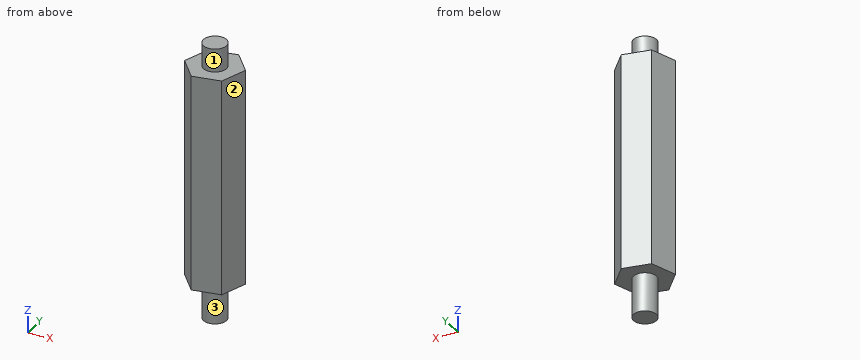
```python
from build123d import *

# Parameters (mm, degrees)
F0_R     = 1.5
F1_DEPTH = 28
F2_DEPTH = 5
F3_R     = 1.5
F4_DEPTH = 3


with BuildPart() as f1:
    # F0 (on Top) → F1 (new body)
    with BuildSketch(Plane.XY):
        Polygon((2.413244, -2.721443), (3.563461, 0.729209), (1.150217, 3.450652), (-2.413244, 2.721443), (-3.563461, -0.729209), (-1.150217, -3.450652), align=None)
        Circle(F0_R, mode=Mode.SUBTRACT)
        Circle(F0_R)
    extrude(amount=F1_DEPTH)

    # F0 (on Top) → F2 (join)
    with BuildSketch(Plane.XY):
        Circle(F0_R)
    extrude(amount=-F2_DEPTH)

    # F3 (on face) → F4 (join)
    with BuildSketch(Plane.XY.offset(28)):
        Circle(F3_R)
    extrude(amount=F4_DEPTH)


solid = f1.part
```
Design review of the part built by this model. Coordinates are the model's own, in mm. Face numbers are marked on the shaded views. A direction names the side the tool comes from. Give positions to 0.01 mm unless a question says otherwise; leave off trailing zeros. Order: outer loops, then holes, each group sorted by start corner. A loop starts at its lowest first (then second) coordinate and runs counter-clockwise, first axis right, second up. Notation, with made-up numbers: (-19.5, -33.75) -> (-4.5, -33.75) arc R18 cw to (-4.5, -3.75) -> close; hole circle Ø8 at (6.25, 51). An arc over 180 degrees is marked (long way). Write each question's results on one line, items separated by ' | '. Start each with the question number.
Q1. Add section C-C on z = 9.5. Give the boundary of the cut face in (x, y).
Q2. For pin 1 (2 mm diameter, centred on y = 1, z = 8.5, fed in from -X); pin 2 (3 mm diameter, centred on x = -2.5, y = 2, fed in from -Z), all flat-tipped, find the tip position at first contact; note any pin that passes through.
Q3. Wall thickness on L1, parallel to Z at x = 0.5, y = 3.25; L2, parallel to X at y = -1.75, z = 15; L3, parallel to Y at x = 1.75, z = 17: over which ranges is each line inside the solid? List them lowest first. Write a range as from..to.
Q4. Machinability: for the marked faces 1, 2 and 3, which of the approach directions +Z, -Z, +X, -X, +Y, -Y give a long, thin tool a straight path to every point of the face, cutting with its end or side? Answer none if there is none.
Q5. Add section D-D on y = -2. Give the boundary of the cut face in (x, z).
Q6. Add section A-A on x = -0.5. Give the boundary of the cut face in (y, z).
Q7. Add section B-B on y = 0. Give the boundary of the cut face in (x, z), and give its area (3 significant figures).
Found:
1) outline: (-3.56, -0.73) -> (-1.15, -3.45) -> (2.41, -2.72) -> (3.56, 0.73) -> (1.15, 3.45) -> (-2.41, 2.72) -> close
2) pin 1: stops at x = -3.32 | pin 2: stops at z = 0
3) L1: z = 0..28 | L2: x = -2.66..2.74 | L3: y = -2.86..2.77
4) face 1: +Z | face 2: +Z, -Z, +X, -Y | face 3: -Z
5) outline: (-2.44, 0) -> (2.65, 0) -> (2.65, 28) -> (-2.44, 28) -> close
6) outline: (-3.32, 0) -> (-1.41, 0) -> (-1.41, -5) -> (1.41, -5) -> (1.41, 0) -> (3.11, 0) -> (3.11, 28) -> (1.41, 28) -> (1.41, 31) -> (-1.41, 31) -> (-1.41, 28) -> (-3.32, 28) -> close
7) outline: (-3.32, 0) -> (-1.5, 0) -> (-1.5, -5) -> (1.5, -5) -> (1.5, 0) -> (3.32, 0) -> (3.32, 28) -> (1.5, 28) -> (1.5, 31) -> (-1.5, 31) -> (-1.5, 28) -> (-3.32, 28) -> close | area: 210 mm2
